CAD build for the part. Positions are in the model's coordinates, mm. Give positions to 0.01 mm unless a question says otherwise; leave off trailing zeros. Write each loop counter-clockwise with the first axis right and the second up, starting at its lowest first coordinate (ties: lowest second). Pieces come first, ordered by that corner, then holes. Notation, with made-up numbers: (-10.75, 77) -> (36.25, 77) arc R20 cw to (36.25, 106) -> close; hole circle Ø7 at (-37, 1). An arc over 180 degrees is marked (long way). Answer as a JSON object with one key per item and string values.
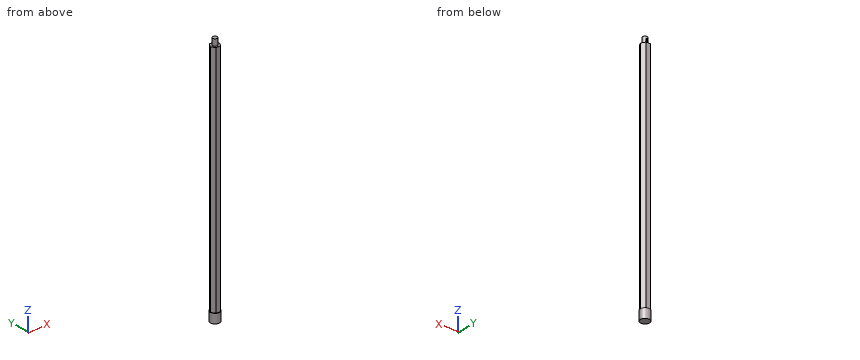
```python
from build123d import *

# Parameters (mm, degrees)
EXTRUDE_1_DEPTH     = 250
SKETCH_2_R          = 2.5
EXTRUDE_2_DEPTH     = 10
SKETCH_3_R          = 5
EXTRUDE_3_DEPTH     = 10
SKETCH_4_W          = 2
SKETCH_4_H          = 1.835573614
CUT_EXTRUDE_1_DEPTH = 10
EXTRUDE_START       = -5
SKETCH_6_R          = 2.5
EXTRUDE_5_DEPTH     = 5
SKETCH_9_R          = 2.5
EXTRUDE_7_DEPTH     = 5
SKETCH_10_R         = 2.5
CUT_EXTRUDE_3_DEPTH = 3
CUT_EXTRUDE_START   = -3
SKETCH_11_R         = 2.5
CUT_EXTRUDE_4_DEPTH = 3
EXTRUDE_START_2     = -10
SKETCH_12_R         = 5
EXTRUDE_8_DEPTH     = 10
SKETCH_14_R         = 2.5
EXTRUDE_10_DEPTH    = 1


with BuildPart() as part:
    # 草图1 → 凸台-拉伸1 (new body)
    with BuildSketch(Plane.XY):
        Polygon((5, 0), (2.5, 4.330127019), (-2.5, 4.330127019), (-5, 0), (-2.5, -4.330127019), (2.5, -4.330127019), align=None)
    extrude(amount=EXTRUDE_1_DEPTH)

    # 草图2 → 凸台-拉伸2 (add)
    with BuildSketch(Plane.XY.offset(250)):
        Circle(SKETCH_2_R)
    extrude(amount=EXTRUDE_2_DEPTH)

    # 草图3 → 凸台-拉伸3 (add)
    with BuildSketch(Plane(origin=(0, 0, 0), x_dir=(-1, 0, 0), z_dir=(0, 0, -1))):
        Circle(SKETCH_3_R)
    extrude(amount=EXTRUDE_3_DEPTH)

    # 草图4 → 切除-拉伸1 (cut)
    with BuildSketch(Plane.XY.offset(260)):
        with Locations((0, 2.417786807)):
            Rectangle(SKETCH_4_W, SKETCH_4_H)
    extrude(amount=-CUT_EXTRUDE_1_DEPTH, mode=Mode.SUBTRACT)

    # 草图6 → 凸台-拉伸5 (add)
    with BuildSketch(Plane.XY.offset(260).offset(EXTRUDE_START)):
        with Locations(Location((0, 0, 0), (0, 0, 113.578178478))):
            Circle(SKETCH_6_R)
    extrude(amount=EXTRUDE_5_DEPTH)

    # 草图9 → 凸台-拉伸7 (add)
    with BuildSketch(Plane(origin=(0, 0, -10), x_dir=(-1, 0, 0), z_dir=(0, 0, -1))):
        with Locations(Location((0, 0, 0), (0, 0, 66.421821522))):
            Circle(SKETCH_9_R)
    extrude(amount=-EXTRUDE_7_DEPTH)

    # 草图10 → 切除-拉伸3 (cut)
    with BuildSketch(Plane(origin=(0, 0, -10), x_dir=(-1, 0, 0), z_dir=(0, 0, -1))):
        with Locations(Location((0, 0, 0), (0, 0, 66.421821522))):
            Circle(SKETCH_10_R)
    extrude(amount=-CUT_EXTRUDE_3_DEPTH, mode=Mode.SUBTRACT)

    # 草图11 → 切除-拉伸4 (cut)
    with BuildSketch(Plane.XY.offset(260).offset(CUT_EXTRUDE_START)):
        with Locations(Location((0, 0, 0), (0, 0, 113.578178478))):
            Circle(SKETCH_11_R)
    extrude(amount=CUT_EXTRUDE_4_DEPTH, mode=Mode.SUBTRACT)

    # 草图12 → 凸台-拉伸8 (add)
    with BuildSketch(Plane(origin=(0, 0, -10), x_dir=(-1, 0, 0), z_dir=(0, 0, -1)).offset(EXTRUDE_START_2)):
        Circle(SKETCH_12_R)
    extrude(amount=EXTRUDE_8_DEPTH)

    # 草图14 → 凸台-拉伸10 (add)
    with BuildSketch(Plane.XY.offset(250)):
        Circle(SKETCH_14_R)
    extrude(amount=EXTRUDE_10_DEPTH)


solid = part.part
```
1) Pin check, flat tips, straight feed: pin 1 (0.6 mm diameter, centred on y = 2, z = 252.5, fed in from -X); pin 2 (4 mm diameter, centred on x = 0.5, z = 188, fed in from +Y); pin 3 (2 mm diameter, centred on x = -0.5, z = 253.5, fed in from +Y); pin 4 (6 mm diameter, centred on x = -1.5, y = 3, fed in from +Z). Stop position of each tip, or through.
Model answer:
{"pin 1": "stops at x = -1.83", "pin 2": "stops at y = 4.33", "pin 3": "stops at y = 2.29", "pin 4": "stops at z = 257"}
2) Wall check: probe 1 along Y at (x, z) = (2, 183); probe 2 along Z at (x, y) = (-3.75, -2); probe 3 along Z at (x, y) = (-4, -2). Give the ranges that are in metal, low to high.
Model answer:
{"probe 1": "y = -4.33 to 4.33", "probe 2": "z = -10 to 250", "probe 3": "z = -10 to 0"}
3) Slice it at A-A (z = 39). List the corners of the cut face in (x, y).
Model answer:
{"outline": "(-5, 0) -> (-2.5, -4.33) -> (2.5, -4.33) -> (5, 0) -> (2.5, 4.33) -> (-2.5, 4.33) -> close"}
